Geometry check sheet. Reference: the model listing, model coordinates, mm. Give positions to 0.01 mm unless a question says otherwise; leave off trailing zeros. Write each loop counter-clockwise with the first axis right and the second up, starting at its lowest first coordinate (ties: lowest second). Pieces come first, ordered by that corner, then holes. Notation, with made-up numbers: M 88,-34 L 94,-34 A23 ccw 94,-17 Z; hole C 55,88 d9. An arc over 180 degrees is marked long. Write each question's results on one line, items separated by ' | '.
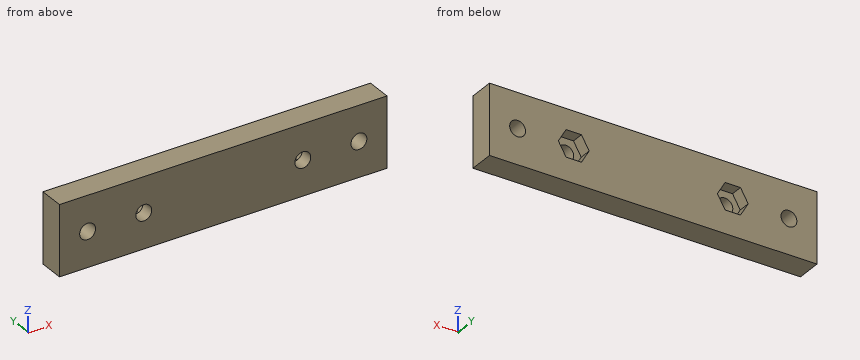
```python
from build123d import *

# Parameters (mm, degrees)
SKETCH1_W           = 70
SKETCH1_H           = 15
BOSS_EXTRUDE1_DEPTH = 5.4
CUT_EXTRUDE1_DEPTH  = 2.6
SKETCH4_R           = 1.7
CUT_EXTRUDE3_DEPTH  = 5.4


with BuildPart() as part:
    # Sketch1 → Boss-Extrude1 (new body)
    with BuildSketch(Plane(origin=(0, 0, 0), x_dir=(1, 0, 0), z_dir=(0, 1, 0))):
        Rectangle(SKETCH1_W, SKETCH1_H)
    extrude(amount=BOSS_EXTRUDE1_DEPTH)

    # Sketch2 → Cut-Extrude1 (cut)
    with BuildSketch(Plane(origin=(0, 5.4, 0), x_dir=(1, 0, 0), z_dir=(0, 1, 0))):
        Polygon((-15.354551733, 2.58658374), (-18.645448267, 2.58658374), (-20.290896534, -0.26341626), (-18.645448267, -3.11341626), (-15.354551733, -3.11341626), (-13.709103466, -0.26341626), align=None)
        Polygon((13.709103466, -0.26341626), (15.354551733, 2.58658374), (18.645448267, 2.58658374), (20.290896534, -0.26341626), (18.645448267, -3.11341626), (15.354551733, -3.11341626), align=None)
    extrude(amount=-CUT_EXTRUDE1_DEPTH, mode=Mode.SUBTRACT)

    # Sketch4 → Cut-Extrude3 (cut)
    with BuildSketch(Plane(origin=(0, 5.4, 0), x_dir=(1, 0, 0), z_dir=(0, 1, 0))):
        with Locations(Location((-29, 0, 0), (0, 0, 270))):
            Circle(SKETCH4_R)
        with Locations(Location((-17, 0, 0), (0, 0, 270))):
            Circle(SKETCH4_R)
        with Locations(Location((17, 0, 0), (0, 0, 270))):
            Circle(SKETCH4_R)
        with Locations(Location((29, 0, 0), (0, 0, 270))):
            Circle(SKETCH4_R)
    extrude(amount=-CUT_EXTRUDE3_DEPTH, mode=Mode.SUBTRACT)


solid = part.part
```
Q1. Depth check by flat-ended pin: P1, Ø2, axis at x = 20.5, z = 5, coming from the -Y side; P2, Ø2, axis at x = -17, z = 0, coming from the +Y side. Enter the tip coordinate at first touch or a pass-through.
Answer key:
P1: stops at y = 0 | P2: passes through
Q2. Section check B-B (x = 29). Enter the section's corners in (y, z), then the cut area to 3 significant figures.
Answer key:
outline: M 0,-7.5 L 5.4,-7.5 L 5.4,-1.7 L 0,-1.7 Z; M 0,1.7 L 5.4,1.7 L 5.4,7.5 L 0,7.5 Z | area: 62.6 mm2
Q3. Material ranges on probe 1 along X at (y, z) = (2.15, 0); probe 2 along X at (y, z) = (1.95, 0.5); probe 3 along X at (y, z) = (2.95, 2.5), recorded low to high. Write a range as [from, to].
Answer key:
probe 1: x = [-35, -30.7], [-27.3, -18.7], [-15.3, 15.3], [18.7, 27.3], [30.7, 35] | probe 2: x = [-35, -30.62], [-27.38, -18.62], [-15.38, 15.38], [18.62, 27.38], [30.62, 35] | probe 3: x = [-35, -19], [-15, 15], [19, 35]
Q4. Section check A-A (y = 4.4). Enter the section's corners in (x, z).
Answer key:
outline: M -35,-7.5 L 35,-7.5 L 35,7.5 L -35,7.5 Z; hole C -29,0 d3.4; hole M -20.29,0.26 L -18.65,-2.59 L -15.35,-2.59 L -13.71,0.26 L -15.35,3.11 L -18.65,3.11 Z; hole M 13.71,0.26 L 15.35,-2.59 L 18.65,-2.59 L 20.29,0.26 L 18.65,3.11 L 15.35,3.11 Z; hole C 29,0 d3.4
Q5. Section check C-C (x = -17). Enter the section's corners in (y, z).
Answer key:
outline: M 0,-7.5 L 5.4,-7.5 L 5.4,-2.59 L 2.8,-2.59 L 2.8,-1.7 L 0,-1.7 Z; M 0,1.7 L 2.8,1.7 L 2.8,3.11 L 5.4,3.11 L 5.4,7.5 L 0,7.5 Z
